Read the model definition and answer for the solid it produces. Units are mm, in the model's axes. Face numbers are marked on the shaded views. A direction names the side the tool comes from. Coordinates: 2 decimals unless noted, no trailing zeros. Order: outer loops, then holes, each group sorted by start corner. A loop starts at its lowest first (then second) coordinate and runs counter-clockwise, first axis right, second up. Notation, with made-up numbers: (51.25, -40) - (107.25, -40) arc R32 cw to (107.25, -8) - close; hole circle Ø1 at (45, -4.75). An arc over 180 degrees is marked (long way). Write item = value, one per line.
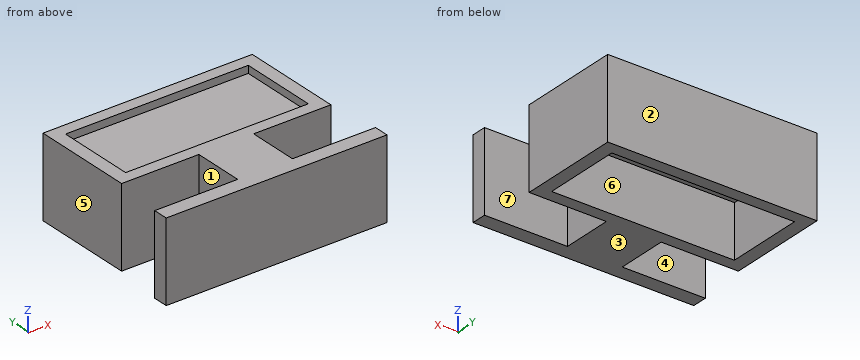
from build123d import *

# Parameters (mm, degrees)
F0_W     = 57.1907274425
F0_H     = 24.536088109
F0_W_2   = 17.1391749755
F0_H_2   = 15.8762889914
F0_H_3   = 0.3608246334
F1_DEPTH = 25
F2_W     = 57.1907274425
F2_H     = 6.2615685165
F3_DEPTH = 25.4


with BuildPart() as f1:
    # F0 (on Top) → F1 (new body)
    with BuildSketch(Plane.XY):
        Polygon((32.7448472381, 16.2371136248), (32.7448472381, 48.3505167067), (-32.7448472381, 48.3505167067), (-32.7448472381, 16.2371136248), (-8.5695888847, 16.2371136248), (8.5695860907, 16.2371136248), align=None)
        with Locations((0, 32.2938151658)):
            Rectangle(F0_W, F0_H, mode=Mode.SUBTRACT)
        with Locations((-1.397e-06, 8.2989691291)):
            Rectangle(F0_W_2, F0_H_2)
        Polygon((34.5489680767, 0.3608246334), (8.5695860907, 0.3608246334), (8.5695860907, 0), (-8.5695888847, 0), (-8.5695888847, 0.3608246334), (-34.5489680767, 0.3608246334), (-34.5489680767, -4.3298969977), (34.5489680767, -4.3298969977), align=None)
        with Locations((-1.397e-06, 0.1804123167)):
            Rectangle(F0_W_2, F0_H_3)
    extrude(amount=F1_DEPTH)

    # F2 (on face) → F3 (join)
    with BuildSketch(Plane(origin=(0, 20.0257711112, 0), x_dir=(-1, 0, 0), z_dir=(0, 1, 0))):
        with Locations((0, 19.563915208)):
            Rectangle(F2_W, F2_H)
    extrude(amount=F3_DEPTH)


solid = f1.part
1) The part is cut by section D-D (z = 18). Determine the outline of the cut face in (x, y), and give its area (3 significant figures).
Returned:
outline = (-34.55, -4.33) - (34.55, -4.33) - (34.55, 0.36) - (8.57, 0.36) - (8.57, 16.24) - (32.74, 16.24) - (32.74, 48.35) - (-32.74, 48.35) - (-32.74, 16.24) - (-8.57, 16.24) - (-8.57, 0.36) - (-34.55, 0.36) - close
area = 2,700 mm^2
2) The part is cut by section A-A (x = -15). Determine the outline of the cut face in (y, z), and give its area (3 significant figures).
Returned:
outline = (-4.33, 0) - (0.36, 0) - (0.36, 25) - (-4.33, 25) - close; (16.24, 0) - (20.03, 0) - (20.03, 16.43) - (44.56, 16.43) - (44.56, 0) - (48.35, 0) - (48.35, 25) - (44.56, 25) - (44.56, 22.69) - (20.03, 22.69) - (20.03, 25) - (16.24, 25) - close
area = 460 mm^2
3) Straight lines are drawn through the part: line 1 along Y through (x, z) = (27.5, 9.25); line 2 along Y through (x, z) = (1, 4.75); line 3 along Y through (x, z) = (31.5, 5.5). For each, find the intervals that lie inside material, in ascending order. Write a range as from..to.
Returned:
line_1 = -4.33..0.36, 16.24..20.03, 44.56..48.35
line_2 = -4.33..20.03, 44.56..48.35
line_3 = -4.33..0.36, 16.24..48.35
4) Flat-ended cylindrical pins translate along their axes: pin 1 Ø10 at (y, z) = (34, 5) entering from -X; pin 2 Ø12 at (x, y) = (13, 30.5) entering from +Z; pin 3 Ø5 at (y, z) = (30.5, 5) entering from +X. Find the tip coordinate at first contact, or state that the pin passes through.
Returned:
pin_1 = -32.74
pin_2 = 22.69
pin_3 = 32.74
5) The part is cut by section C-C (y = 28). Determine the outline of the cut face in (x, z), and give its area (3 significant figures).
Returned:
outline = (-32.74, 0) - (-28.6, 0) - (-28.6, 16.43) - (28.6, 16.43) - (28.6, 0) - (32.74, 0) - (32.74, 25) - (28.6, 25) - (28.6, 22.69) - (-28.6, 22.69) - (-28.6, 25) - (-32.74, 25) - close
area = 566 mm^2
6) The part is cut by section B-B (z = 9.5). Determine the outline of the cut face in (x, y), and give its area (3 significant figures).
Returned:
outline = (-34.55, -4.33) - (34.55, -4.33) - (34.55, 0.36) - (8.57, 0.36) - (8.57, 16.24) - (32.74, 16.24) - (32.74, 48.35) - (-32.74, 48.35) - (-32.74, 16.24) - (-8.57, 16.24) - (-8.57, 0.36) - (-34.55, 0.36) - close; hole (-28.6, 20.03) - (28.6, 20.03) - (28.6, 44.56) - (-28.6, 44.56) - close
area = 1,300 mm^2
7) For the marked faces 4, 5, 6 and 7, determine the directions among +Z, -Z, +X, -X, +Y, -Y from which every point of the face is accessible in a straight line to the end or side of a thin tool.
Returned:
face_4 = +Z, -Z, -X
face_5 = +Z, -Z, -X, +Y
face_6 = -Z
face_7 = +Z, -Z, +X
8) Determine the mould class of the marked faces 1, 2 and 3 for opening direction Y: pulls with the +Y half, pulls with the -Y half, needs draft (parallel to the pull), parting line crosses it, or undercut.
Returned:
face_1 = undercut
face_2 = pulls with the +Y half
face_3 = needs draft
